```python
from build123d import *

# Parameters (mm, degrees)
SKETCH_W            = 25.4
SKETCH_H            = 52
SKETCH_R            = 3.375
PAD_DEPTH           = 3
PAD001_DEPTH        = 62
POCKET_DEPTH        = 59
SKETCH004_W         = 22
SKETCH004_H         = 54
POCKET001_DEPTH     = 5
FILLET_R            = 3
PAD002_DEPTH        = 2
LINEARPATTERN_COUNT = 3
LINEARPATTERN_PITCH = 25
FILLET001_R         = 1


with BuildPart() as part:
    # Sketch → Pad (new body)
    with BuildSketch(Plane.XZ):
        with Locations((0, 26)):
            Rectangle(SKETCH_W, SKETCH_H)
        with Locations((0, 39)):
            Circle(SKETCH_R, mode=Mode.SUBTRACT)
        with Locations((0, 13)):
            Circle(SKETCH_R, mode=Mode.SUBTRACT)
    extrude(amount=PAD_DEPTH)

    # Sketch001 → Pad001 (join)
    with BuildSketch(Plane.XY):
        with BuildLine():
            Line((-51, -5), (-51, -16))
            ThreePointArc((-51, -16), (-49.535534, -19.535534), (-46, -21))
            Line((-46, -21), (-13, -21))
            ThreePointArc((-13, -21), (-9.464466, -19.535534), (-8, -16))
            Line((-8, -16), (-8, 0))
            Line((-46, 0), (-8, 0))
            ThreePointArc((-46, 0), (-49.535534, -1.464466), (-51, -5))
        make_face()
    extrude(amount=PAD001_DEPTH)

    # Sketch003 → Pocket (cut)
    with BuildSketch(Plane(origin=(0, 0, 62), x_dir=(-1, 0, 0), z_dir=(0, 0, 1))):
        with BuildLine():
            Line((49, 15.5), (49, 10.5))
            ThreePointArc((34.5, 3), (42.662414, 4.986), (49, 10.5))
            Line((24.5, 3), (34.5, 3))
            ThreePointArc((10, 10.5), (16.337586, 4.986), (24.5, 3))
            Line((10, 10.5), (10, 15.5))
            ThreePointArc((49, 15.5), (29.5, 18), (10, 15.5))
        make_face()
    extrude(amount=-POCKET_DEPTH, mode=Mode.SUBTRACT)

    # Sketch004 (on Face11 of Pocket) → Pocket001 (cut)
    with BuildSketch(Plane.XZ.offset(21)):
        with Locations((-29.5, 35)):
            Rectangle(SKETCH004_W, SKETCH004_H)
    extrude(amount=-POCKET001_DEPTH, mode=Mode.SUBTRACT)

    # Fillet
    fillet_edges = [part.edges().sort_by_distance(p)[0] for p in [
        (12.7, -1.5, 52),
        (12.7, -1.5, 0),
    ]]
    fillet(fillet_edges, radius=FILLET_R)

    # Sketch005 → Pad002 (join)
    with BuildSketch(Plane.XY):
        Polygon((-8, -16), (-8, -3), (5, -3), align=None)
    pad002 = extrude(amount=PAD002_DEPTH)

    # LinearPattern: Pad002 ×3
    with Locations(*[(0, 0, i * LINEARPATTERN_PITCH) for i in range(1, LINEARPATTERN_COUNT)]):
        add(pad002)

    # Fillet001
    fillet001_edges = [part.edges().sort_by_distance(p)[0] for p in [
        (-8, -3, 38.5),
        (-8, -3, 13.5),
        (-18.5, -21, 35),
        (-29.5, -21, 8),
        (-40.5, -21, 35),
        (-40.5, -19.106666, 62),
        (-18.5, -19.106666, 62),
        (-40.5, -17.213332, 35),
        (-29.5, -18, 8),
        (-18.5, -17.213332, 35),
        (-14.225957, -16.475944, 62),
        (-10, -13, 62),
        (-16.337586, -4.986, 62),
        (-29.5, -3, 62),
        (-42.662414, -4.986, 62),
        (-49, -13, 62),
        (-44.774043, -16.475944, 62),
    ]]
    fillet(fillet001_edges, radius=FILLET001_R)


solid = part.part
```
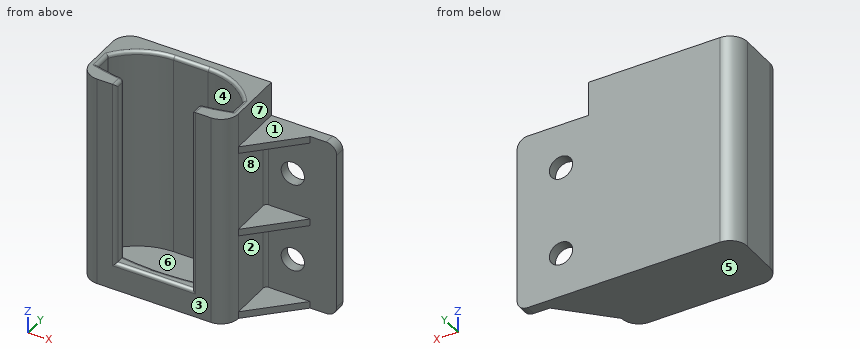
Geometry: final body of the model. Coordinates: model frame, mm. Face numbers are marked on the shaded views. A direction names the side the tool comes from. Round coordinates to 2 decimals unless told otherwise and drop trailing zeros. Order: outer loops, then holes, each group sorted by start corner. A loop starts at its lowest first (then second) coordinate and runs counter-clockwise, first axis right, second up. Notation, with made-up numbers: M 24.5,53 L 64.5,53 A22 cw 64.5,74 Z; hole C 74.5,-13.75 d10. An arc over 180 degrees is marked long. Use one line per item in the form item = value. Start each with the question number.
Q1. Material intervals for line 1 (Z direction, x = 0, y = -1.6) (3 decimals); line 2 (X direction, y = -13.75, z = 38); line 3 (Z direction, x = -40.5, y = -11.75), sorted ascending. Write a range as [from, to].
Q2. Pin query (flat end, axial travel): pin 1 Ø4 at (x, z) = (0, 39) entering from +Y; pin 2 Ø6 at (y, z) = (-9, 11) entering from +X; pin 3 Ø11 at (y, z) = (-9.5, 56.5) entering from +X; pin 4 Ø4.5 at (x, y) = (-31.5, -13) entering from +Z. Return the tip coordinate at first contact, or that it passes through.
Q3. Mould query, pull axis Z, two halves, no side actions, for the marked faces 6, 7 and 8. Classes: +Z half, -Z half, draft (parallel to the pull), parting line (faces both ways), or undercut.
Q4. Cut plane B-B (x = 0). Return loops of the section in (y, z) (3 decimals), and give its area (4 significant figures).
Q5. Cut plane A-A (z = 39). Return loops of the section in (x, y) (3 decimals), and give its area (3 significant figures).
Q6. Access query for the marked faces 1, 2, 3, 4 and 5. Directions: +Z, -Z, +X, -X, +Y, -Y. A direction counts if a zero-diameter tool reaches every point of the face in a straight line with its end or side. Return the directions, or none.
Q7. Cut plane C-C (y = -12.75). Return loops of the section in (x, z).
Q8. Cut plane D-D (z = 18). Return loops of the section in (x, y) (3 decimals).
Geometry results:
q1.line_1 = [0, 9.625], [16.375, 35.625], [42.375, 52]
q1.line_2 = [-51, -49], [-10, -8]
q1.line_3 = [0, 3]
q2.pin_1 = through
q2.pin_2 = -8
q2.pin_3 = 1.66
q2.pin_4 = 3
q3.face_6 = +Z half
q3.face_7 = draft
q3.face_8 = undercut
q4.outline = M -8,0 L 0,0 L 0,9.625 L -3,9.625 L -3,2 L -8,2 Z; M -8,25 L -3,25 L -3,16.375 L 0,16.375 L 0,35.625 L -3,35.625 L -3,27 L -8,27 Z; M -8,50 L -3,50 L -3,42.375 L 0,42.375 L 0,52 L -8,52 Z
q4.area = 145.5 mm^2
q5.outline = M -51,-16 A5 ccw -46,-21 L -41.5,-21 A1 ccw -40.5,-20 L -40.5,-18.075 A1 ccw -41.347,-17.087 A77.3 cw -49,-15.5 L -49,-10.5 A17.767 cw -34.5,-3 L -24.5,-3 A17.767 cw -10,-10.5 L -10,-15.5 A77.3 cw -17.653,-17.087 A1 ccw -18.5,-18.075 L -18.5,-20 A1 ccw -17.5,-21 L -13,-21 A5 ccw -8,-16 L -8,-4 A1 cw -7,-3 L -3.375,-3 L -3.375,0 L -46,0 A5 ccw -51,-5 Z; M 3.375,-3 L 12.7,-3 L 12.7,0 L 3.375,0 Z
q5.area = 369 mm^2
q6.face_1 = +Z, +X, +Y, -Y
q6.face_2 = +X, -Y
q6.face_3 = +Z, -Z, +X, -X, -Y
q6.face_4 = +Z
q6.face_5 = -Z, +X, -X, +Y, -Y
q7.outline = M -51,0 L -4.75,0 L -4.75,2 L -8,2 L -8,25 L -4.75,25 L -4.75,27 L -8,27 L -8,50 L -4.75,50 L -4.75,52 L -8,52 L -8,62 L -9,62 A1 ccw -10,61 L -10,3 L -49,3 L -49,61 A1 ccw -50,62 L -51,62 Z
q8.outline = M -51,-16 A5 ccw -46,-21 L -41.5,-21 A1 ccw -40.5,-20 L -40.5,-18.075 A1 ccw -41.347,-17.087 A77.3 cw -49,-15.5 L -49,-10.5 A17.767 cw -34.5,-3 L -24.5,-3 A17.767 cw -10,-10.5 L -10,-15.5 A77.3 cw -17.653,-17.087 A1 ccw -18.5,-18.075 L -18.5,-20 A1 ccw -17.5,-21 L -13,-21 A5 ccw -8,-16 L -8,-4 A1 cw -7,-3 L 12.7,-3 L 12.7,0 L -46,0 A5 ccw -51,-5 Z
